The listing builds one solid part. Answer for the finished solid, in the listing's coordinates (mm). Face numbers are marked on the shaded views. Give positions to 0.01 mm unless a question says otherwise; leave off trailing zeros. Order: outer loops, then holes, each group sorted by start corner. A loop starts at its lowest first (then second) coordinate and runs counter-clockwise, first axis right, second up. Notation, with made-up numbers: (23, 20) -> (31, 20) arc R23 ccw to (31, 30) -> close; hole circle Ø11 at (73.5, 4.5). An arc over 180 degrees is marked (long way). Answer as a JSON object with one key per item and string values. Group by question number.
```python
from build123d import *

# Parameters (mm, degrees)
SKETCH001_R           = 2
POCKET_DEPTH          = 317.933954
POCKET_DEPTH_BACK     = 312.533954
POLARPATTERN_COUNT    = 4
POCKET001_DEPTH       = 1
POLARPATTERN001_COUNT = 4


with BuildPart() as part:
    # Sketch → Revolution (revolve)
    with BuildSketch(Plane.YZ):
        Polygon((-37.6, 0), (-48, 0), (-48, 3.2), (-46.6, 4.4), (-46.6, 6), (-48, 7.2), (-48, 11.2), (-46.6, 12.4), (-46.6, 16), (-48, 17.2), (-48, 18.4), (-53.3, 18.4), (-53.3, 21.4), (-43, 21.4), (-39.5, 18.4), (-39.5, 13.4), (-37.6, 13.4), align=None)
    revolve(axis=Axis((0, 0, 0), (0, 0, 1)))

    # Sketch001 (on Face16 of Revolution) → Pocket (cut, two sides)
    with BuildSketch(Plane(origin=(0, 0, 13.4), x_dir=(0, -1, 0), z_dir=(0, 0, 1))) as pocket_sk:
        with Locations((0, 39.95)):
            Circle(SKETCH001_R)
    pocket = extrude(amount=-POCKET_DEPTH, mode=Mode.SUBTRACT) + extrude(pocket_sk.sketch, amount=POCKET_DEPTH_BACK, mode=Mode.SUBTRACT)

    # PolarPattern: Pocket ×4 about axis
    polarpattern_axis = Axis((0, 0, 13.4), (0, 0, 1))
    for i in range(1, POLARPATTERN_COUNT):
        add(pocket.rotate(polarpattern_axis, i * 360 / POLARPATTERN_COUNT), mode=Mode.SUBTRACT)

    # Sketch002 (on Face11 of PolarPattern) → Pocket001 (cut)
    with BuildSketch(Plane(origin=(0, 0, 13.4), x_dir=(0, -1, 0), z_dir=(0, 0, 1))):
        with BuildLine():
            Line((-41.95, 0), (0, 0))
            Line((0, 0), (-36.329766, 20.975))
            ThreePointArc((-36.329766, 20.975), (-40.520588, 10.857459), (-41.95, 0))
        make_face()
    pocket001 = extrude(amount=POCKET001_DEPTH, mode=Mode.SUBTRACT)

    # PolarPattern001: Pocket001 ×4 about axis
    polarpattern001_axis = Axis((0, 0, 13.4), (0, 0, 1))
    for i in range(1, POLARPATTERN001_COUNT):
        add(pocket001.rotate(polarpattern001_axis, i * 360 / POLARPATTERN001_COUNT), mode=Mode.SUBTRACT)


solid = part.part
```
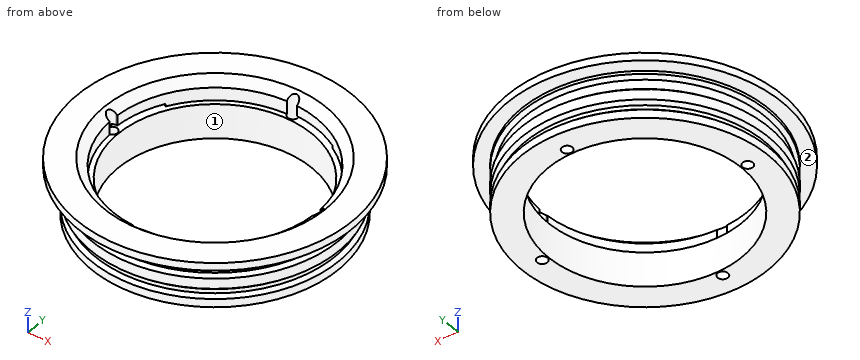
(1) For a pull along Y with two mould halves and no side action, classify the marked faces 1 and 2 as +Y half, -Y half, draft (parallel to the pull), parting line (faces both ways), or undercut.
(2) A cutting plane is placed at A-A (z = 8.5). Determine the outline of the cut face in (x, y).
(3) Find the intervals of material crossed by line 1 along X through (y, z) = (0, 9.75); line 2 along Y through (x, z) = (1, 5.25); line 3 along Z through (x, y) = (-17, -43.5), in increasing order. Write a range as [from, to].
(4) Flat-ended cylindrical pins translate along their axes: pin 1 Ø25 at (x, y) = (15, -14.5) entering from +Z; pin 2 Ø8 at (x, z) = (-31.5, 12) entering from -Y; pin 3 Ø5 at (x, y) = (-39.95, 0) entering from +Z; pin 4 Ø3 at (x, z) = (-25, 12) entering from +Y. Find the tip coordinate at first contact, or state that the pin passes through.
Check sheet entries:
{
 "1": {"face 1": "undercut", "face 2": "draft"},
 "2": {"outline": "circle Ø96 at (0, 0); hole circle Ø4 at (-39.95, 0); hole circle Ø75.2 at (0, 0); hole circle Ø4 at (0, -39.95); hole circle Ø4 at (0, 39.95); hole circle Ø4 at (39.95, 0)"},
 "3": {"line 1": "x = [-48, -41.95], [-37.95, -37.6], [37.6, 37.95], [41.95, 48]", "line 2": "y = [-46.59, -41.68], [-38.22, -37.59], [37.59, 38.22], [41.68, 46.59]", "line 3": "z = [0, 4.31], [6.09, 12.31], [16.09, 21.4]"},
 "4": {"pin 1": "passes through", "pin 2": "stops at y = -39.28", "pin 3": "stops at z = 20.93", "pin 4": "stops at y = 41.72"}
}
